Source: CAD feature listing. Evaluate the final solid. Frame: model axes, mm. A direction names the side the tool comes from. Coordinates: 2 decimals unless noted, no trailing zeros. Order: outer loops, then holes, each group sorted by start corner. A loop starts at its lowest first (then second) coordinate and runs counter-clockwise, first axis right, second up. Notation, with made-up numbers: (13.5, 65) -> (43.5, 65) arc R27 cw to (43.5, 93) -> close; hole circle Ø1 at (89.25, 83). An arc over 180 degrees is marked (long way). Write each question's results on one line, items separated by ' | '. Start each with the question number.
Autodesk Inventor part; units mm, degrees
ref_plane "YZ Plane" through (0, 0, 0) normal (1, 0, 0) x (0, 1, 0)
ref_plane "XZ Plane" through (0, 0, 0) normal (0, 1, 0) x (-1, 0, 0)
ref_plane "XY Plane" through (0, 0, 0) normal (0, 0, 1) x (1, 0, 0)
sketch "Sketch1" plane through (0, 0, 0) normal (0, 1, 0) x (-1, 0, 0)
  line L0 (-8.128, 10.16) -> (8.128, 10.16)
  line L1 (8.128, 10.16) -> (8.128, -10.16)
  line L2 (8.128, -10.16) -> (-8.128, -10.16)
  line L3 (-8.128, -10.16) -> (-8.128, 10.16)
  line L4 (-8.128, 10.16) -> (8.128, -10.16) construction
  line L5 (8.128, 10.16) -> (-8.128, -10.16) construction
  point P0 (0, 0)
  dimension "d0" = 20.32
  dimension "d1" = 16.256
extrude "Extrusion1" add sketch "Sketch1" along normal mid plane 12.2492
sketch "Sketch3" plane through (0, -6.1246, 0) normal (0, -1, 0) x (1, 0, 0)
  line L0 (-5.203, 2.905) -> (5.203, 2.905)
  line L1 (5.203, 2.905) -> (5.203, -2.905)
  line L2 (5.203, -2.905) -> (-5.203, -2.905)
  line L3 (-5.203, -2.905) -> (-5.203, 2.905)
  line L4 (-5.203, 2.905) -> (5.203, -2.905) construction
  line L5 (5.203, 2.905) -> (-5.203, -2.905) construction
  point P0 (0, 0)
  dimension "d4" = 5.81
  dimension "d5" = 10.406
extrude "Extrusion2" cut sketch "Sketch3" against normal through all
sketch "Sketch4" plane through (0, -6.1246, 0) normal (0, -1, 0) x (1, 0, 0)
  line L0 (-4.9149, 6.985) -> (4.9149, 6.985) construction
  line L1 (4.9149, 6.985) -> (4.9149, 4.1402) construction
  line L2 (4.9149, 4.1402) -> (-4.9149, 4.1402) construction
  line L3 (-4.9149, 4.1402) -> (-4.9149, 6.985) construction
  line L4 (-4.9149, 6.985) -> (4.9149, 4.1402) construction
  line L5 (4.9149, 6.985) -> (-4.9149, 4.1402) construction
  line L6 (5.1649, 7.235) -> (-5.1649, 7.235)
  line L7 (-5.1649, 7.235) -> (-5.1649, 3.8902)
  line L8 (-5.1649, 3.8902) -> (5.1649, 3.8902)
  line L9 (5.1649, 3.8902) -> (5.1649, 7.235)
  point P0 (0, 0)
  point P1 (0, 5.5626)
  dimension "d8" = 2.8448
  dimension "d9" = 9.8298
  dimension "d10" = 6.985
  dimension "d13" = 0.25
extrude "Extrusion3" cut sketch "Sketch4" against normal blind 2.6099
mirror "Mirror1" about plane through (0, 0, 0) normal (0, 0, 1) of "Extrusion3"
sketch "Sketch5" plane through (0, -6.1246, 0) normal (0, -1, 0) x (1, 0, 0)
  line L0 (-5.203, -2.905) -> (-5.203, 2.905)
  line L1 (-5.203, 1.5875) -> (-6.7905, 1.5875)
  line L2 (-6.7905, 1.5875) -> (-6.7905, -1.5875)
  line L3 (-6.7905, -1.5875) -> (-5.203, -1.5875)
  line L4 (-5.203, -1.5875) -> (-5.203, 1.5875)
  point P0 (0, 0)
  point P1 (-6.7905, 0)
  dimension "d14" = 1.5875
  dimension "d15" = 3.175
extrude "Extrusion4" add sketch "Sketch5" along normal blind 2.2669
mirror "Mirror2" about plane through (0, 0, 0) normal (1, 0, 0) of "Extrusion4"
sketch "Sketch6" plane through (0, -6.1246, 0) normal (0, -1, 0) x (1, 0, 0)
  line L0 (-5.1649, 7.235) -> (5.1649, 7.235)
  line L1 (1.5875, 7.235) -> (-1.5875, 7.235)
  line L2 (-1.5875, 7.235) -> (-1.5875, 8.8225)
  line L3 (-1.5875, 8.8225) -> (1.5875, 8.8225)
  line L4 (1.5875, 8.8225) -> (1.5875, 7.235)
  point P0 (0, 0)
  point P1 (0, 7.235)
  dimension "d18" = 1.5875
  dimension "d19" = 3.175
extrude "Extrusion5" add sketch "Sketch6" along normal up to surface (2.2669 mm away)
mirror "Mirror3" about plane through (0, 0, 0) normal (0, 0, 1) of "Extrusion5"
sketch "Sketch7" plane through (0, -6.1246, 0) normal (0, -1, 0) x (1, 0, 0)
  line L0 (5.203, -2.905) -> (5.203, 2.905)
  line L1 (5.203, 2.905) -> (-5.203, 2.905)
  line L2 (-5.203, 2.905) -> (-5.203, 3.159)
  line L3 (-5.203, 3.159) -> (5.203, 3.159)
  line L4 (5.203, 3.159) -> (5.203, 2.905)
  point P0 (0, 0)
  point P1 (-5.203, 3.032)
  dimension "d22" = 0.254
extrude "Extrusion6" add sketch "Sketch7" along normal blind 0.62
mirror "Mirror4" about plane through (0, 0, 0) normal (0, 0, 1) of "Extrusion6"
properties part number "magnet_jig"
(1) Reachability of faces 5 (the flat face through (0, -3.515, 6)), 6 (the flat face through (-6, -7, 1.588)), 7 (the flat face through (5.203, -1, 0)), 8 (the flat face through (0, -7, -8.822)) from +Z, -Z, +X, -X, +Y, -Y: full face, straight path, thin tool, end or side. Return the list, or none.
(2) First-contact query: P1, Ø3, axis at x = 3.5, z = -7, coming from the -Y side; P2, Ø5.5, axis at x = 1, y = -7, coming from the +Z side; P3, Ø4, axis at x = 2.5, z = 4.5, coming from the -Y side; P4, Ø0.5, axis at x = 5.5, y = -7.5, coming from the +Z side. Flat tips, straight axial feed; report the tip coordinate or a pass-through.
(3) Section D-D on y = -5.75. Return the cut outline in (x, z) (3 decimals).
(4) Section C-C on x = 2.5. Return the cut outline in (y, z) (3 decimals), then the cut area to 3 significant figures.
(5) Draft query along Z for faces 1 (the flat face through (6, -8.392, 0)), 2 (the flat face through (6, -7, 1.588)), 3 (the flat face through (0, -5, 3.89)), 4 (the flat face through (5.165, -5, -6)). Return one class per face: released by +Z, released by -Z, zero draft, split by the parting line, or undercut.
(6) Section A-A on z = -2.5. Return the cut outline in (x, y), then the cut area to 3 significant figures.
(7) Section B-B on y = 1. Return the cut outline in (x, z) (3 decimals).
(8) Line query: L1, parallel to Z at x = 2.25, y = -4.25 (3 decimals); L2, parallel to X at y = 1, z = 2.5; L3, parallel to Z at x = 0, y = 0.5 (3 decimals). Output: solid intervals per line, ascending.
Results list:
1) face 5: -Y | face 6: +Z, +X, -X, -Y | face 7: +Y, -Y | face 8: -Z, +X, -X, -Y
2) P1: stops at y = -6.12 | P2: stops at z = 10.16 | P3: stops at y = -6.74 | P4: stops at z = 1.59
3) outline: (-8.128, -10.16) -> (8.128, -10.16) -> (8.128, 10.16) -> (-8.128, 10.16) -> close; hole (-5.203, -2.905) -> (5.203, -2.905) -> (5.203, 2.905) -> (-5.203, 2.905) -> close; hole (-5.165, -7.235) -> (5.165, -7.235) -> (5.165, -3.89) -> (-5.165, -3.89) -> close; hole (-5.165, 3.89) -> (5.165, 3.89) -> (5.165, 7.235) -> (-5.165, 7.235) -> close
4) outline: (-6.745, -3.159) -> (-6.125, -3.159) -> (-6.125, -3.89) -> (-3.515, -3.89) -> (-3.515, -7.235) -> (-6.125, -7.235) -> (-6.125, -10.16) -> (6.125, -10.16) -> (6.125, -2.905) -> (-6.745, -2.905) -> close; (-6.745, 2.905) -> (6.125, 2.905) -> (6.125, 10.16) -> (-6.125, 10.16) -> (-6.125, 7.235) -> (-3.515, 7.235) -> (-3.515, 3.89) -> (-6.125, 3.89) -> (-6.125, 3.159) -> (-6.745, 3.159) -> close | area: 161 mm²
5) face 1: zero draft | face 2: released by +Z | face 3: undercut | face 4: undercut
6) outline: (-8.13, -6.12) -> (-5.2, -6.12) -> (-5.2, 6.12) -> (-8.13, 6.12) -> close; (5.2, -6.12) -> (8.13, -6.12) -> (8.13, 6.12) -> (5.2, 6.12) -> close | area: 71.7 mm²
7) outline: (-8.128, -10.16) -> (8.128, -10.16) -> (8.128, 10.16) -> (-8.128, 10.16) -> close; hole (-5.203, -2.905) -> (5.203, -2.905) -> (5.203, 2.905) -> (-5.203, 2.905) -> close
8) L1: z = -10.16 to -7.235, -3.89 to -2.905, 2.905 to 3.89, 7.235 to 10.16 | L2: x = -8.13 to -5.2, 5.2 to 8.13 | L3: z = -10.16 to -2.905, 2.905 to 10.16
